Design review of the part built by this model. Coordinates are the model's own, in mm. A direction names the side the tool comes from. Coordinates: 2 decimals unless noted, no trailing zeros. Write each loop counter-clockwise with the first axis right and the second up, starting at its lowest first coordinate (ties: lowest second). Pieces come first, ordered by that corner, then holes. Notation, with made-up numbers: (-13, 17) -> (43, 17) arc R37 cw to (43, 56) -> close; hole circle Ø5 at (39, 8.5). An arc over 180 degrees is marked (long way). Answer in a Markdown table with one row per item. Add a question column.
Item 1: Take a section at B-B, the plane x = -2.5. Write out the cut boundary in (y, z), and give its area (3 significant figures).
Item 2: Take a section at D-D, the plane y = 23. Write out the cut boundary in (x, z), and give its area (3 significant figures).
Item 3: Take a section at A-A, the plane y = 38. Give the number of separate pieces and of enclosed holes in the cut face, and give its area (3 significant figures).
Item 4: To check wall thickness, follow line 1 (Z direction, x = 13.5, y = 36); line 2 (Y direction, x = -2.5, z = -1.65); line 3 (X direction, y = 32, z = -53). State the ranges of each line that lie inside material, in increasing order.
Item 5: Draft analysis for pull direction Z (two halves, no side actions). For faces 4 (the face through (15, 24, 0)), 5 (the face through (19.3, 35.1, -143.9)), 6 (the face through (-2.33, 39.29, -1.52)), state which applies: released by +Z, released by -Z, zero draft, split by the parting line, or undercut.
Item 6: For faces 1 (the face through (15, 20, -92)), 2 (the face through (15, 30, -97)), 3 (the face through (15, 30, -87)), list the 3-axis set-ups (+Z, -Z, +X, -X, +Y, -Y) from which the entire face can be reached by the end or side of a thin tool; tool diameter is ignored.
Item 7: Take a section at C-C, the plane z = -42. Write out the cut boundary in (x, y).
Item 8: Clearance check with flat-ended pins moving along their axes: P1, Ø16, axis at y = 28.5, z = -86.5, coming from the -X side; P2, Ø1.4, axis at x = 20, z = -142.92, coming from the +Y side; P3, Ø1.5, axis at x = -2, y = 31, coming from the -Z side. State where each tip first meets the part, or that it passes through.
from build123d import *

# Parameters (mm, degrees)
SKETCH1_W               = 30
SKETCH1_H               = 150
BOSS_EXTRUDE1_DEPTH     = 40
CUT_EXTRUDE1_DEPTH      = 159.113883008
CUT_EXTRUDE1_DEPTH_BACK = 30
SKETCH2_W               = 22
SKETCH2_H               = 43
SKETCH4_W               = 22
SKETCH4_H               = 10
CUT_EXTRUDE2_DEPTH      = 20
CUT_EXTRUDE3_DEPTH      = 159.113883008
CUT_EXTRUDE3_DEPTH_BACK = 159.113883008
SKETCH5_W               = 150
SKETCH5_H               = 8
SKETCH6_R               = 1.2
CUT_EXTRUDE4_DEPTH      = 10
SKETCH7_W               = 40
SKETCH7_H               = 32
BOSS_EXTRUDE2_DEPTH     = 3
SKETCH8_R               = 1.3
CUT_EXTRUDE5_DEPTH      = 157.31378698
SKETCH9_W               = 22
SKETCH9_H               = 80
CUT_EXTRUDE6_DEPTH      = 158.318148985


with BuildPart() as part:
    # Sketch1 → Boss-Extrude1 (new body)
    with BuildSketch(Plane(origin=(0, 0, 0), x_dir=(1, 0, 0), z_dir=(0, 1, 0))):
        with Locations((15, 75)):
            Rectangle(SKETCH1_W, SKETCH1_H)
    extrude(amount=BOSS_EXTRUDE1_DEPTH)

    # Sketch2 → Cut-Extrude1 (cut, two sides: drawn at the far end of the back side and taken through both)
    with BuildSketch(Plane(origin=(0, 40, 0), x_dir=(1, 0, 0), z_dir=(0, 1, 0)).offset(-CUT_EXTRUDE1_DEPTH_BACK)):
        with Locations((15, 118.5)):
            Rectangle(SKETCH2_W, SKETCH2_H)
    extrude(amount=CUT_EXTRUDE1_DEPTH + CUT_EXTRUDE1_DEPTH_BACK, mode=Mode.SUBTRACT)

    # Sketch4 → Cut-Extrude2 (cut)
    with BuildSketch(Plane.XZ):
        with Locations((15, -92)):
            Rectangle(SKETCH4_W, SKETCH4_H)
    extrude(amount=-CUT_EXTRUDE2_DEPTH, mode=Mode.SUBTRACT)

    # Sketch5 → Cut-Extrude3 (cut, two sides: drawn at the far end of the back side and taken through both)
    with BuildSketch(Plane.ZY.offset(-CUT_EXTRUDE3_DEPTH_BACK)):
        with Locations((-75, 4)):
            Rectangle(SKETCH5_W, SKETCH5_H)
    extrude(amount=CUT_EXTRUDE3_DEPTH + CUT_EXTRUDE3_DEPTH_BACK, mode=Mode.SUBTRACT)

    # Sketch6 → Cut-Extrude4 (cut)
    with BuildSketch(Plane(origin=(0, 40, 0), x_dir=(1, 0, 0), z_dir=(0, 1, 0))):
        with Locations(Location((10, 142.924700648, 0), (0, 0, 270))):
            Circle(SKETCH6_R)
        with Locations(Location((20, 142.924700648, 0), (0, 0, 270))):
            Circle(SKETCH6_R)
        with Locations(Location((10, 94.924700648, 0), (0, 0, 270))):
            Circle(SKETCH6_R)
        with Locations(Location((20, 94.924700648, 0), (0, 0, 270))):
            Circle(SKETCH6_R)
    extrude(amount=-CUT_EXTRUDE4_DEPTH, mode=Mode.SUBTRACT)

    # Sketch7 → Boss-Extrude2 (add)
    with BuildSketch(Plane.XY):
        with Locations((15, 24)):
            Rectangle(SKETCH7_W, SKETCH7_H)
    extrude(amount=-BOSS_EXTRUDE2_DEPTH)

    # Sketch8 → Cut-Extrude5 (cut, through all)
    with BuildSketch(Plane(origin=(0, 0, -3), x_dir=(-1, 0, 0), z_dir=(0, 0, -1))):
        with Locations((-32.5, 38)):
            Circle(SKETCH8_R)
        with Locations((-32.5, 10)):
            Circle(SKETCH8_R)
        with Locations((2.5, 38)):
            Circle(SKETCH8_R)
        with Locations((2.5, 10)):
            Circle(SKETCH8_R)
    extrude(amount=-CUT_EXTRUDE5_DEPTH, mode=Mode.SUBTRACT)

    # Sketch9 → Cut-Extrude6 (cut, through all)
    with BuildSketch(Plane(origin=(0, 40, 0), x_dir=(1, 0, 0), z_dir=(0, 1, 0))):
        with Locations((15, 47)):
            Rectangle(SKETCH9_W, SKETCH9_H)
    extrude(amount=-CUT_EXTRUDE6_DEPTH, mode=Mode.SUBTRACT)


solid = part.part
Answers:
| question | item | result |
|---|---|---|
| 1 | outline | (8, -3) -> (8.7, -3) -> (8.7, 0) -> (8, 0) -> close; (11.3, -3) -> (36.7, -3) -> (36.7, 0) -> (11.3, 0) -> close; (39.3, -3) -> (40, -3) -> (40, 0) -> (39.3, 0) -> close |
| 1 | area | 80.4 mm^2 |
| 2 | outline | (-5, -3) -> (0, -3) -> (0, -150) -> (30, -150) -> (30, -3) -> (35, -3) -> (35, 0) -> (-5, 0) -> close; hole (4, -140) -> (26, -140) -> (26, -97) -> (4, -97) -> close; hole (4, -87) -> (26, -87) -> (26, -7) -> (4, -7) -> close |
| 2 | area | 1,820 mm^2 |
| 3 | separate pieces | 3 |
| 3 | enclosed holes | 6 |
| 3 | area | 1,790 mm^2 |
| 4 | line 1 | z = -150 to -140, -97 to -87, -7 to 0 |
| 4 | line 2 | y = 8 to 8.7, 11.3 to 36.7, 39.3 to 40 |
| 4 | line 3 | x = 0 to 4, 26 to 30 |
| 5 | face 4 | released by +Z |
| 5 | face 5 | undercut |
| 5 | face 6 | zero draft |
| 6 | face 1 | -Y |
| 6 | face 2 | +Y |
| 6 | face 3 | +Y, -Y |
| 7 | outline | (0, 8) -> (4, 8) -> (4, 40) -> (0, 40) -> close; (26, 8) -> (30, 8) -> (30, 40) -> (26, 40) -> close |
| 8 | P1 | stops at x = 0 |
| 8 | P2 | stops at y = 30 |
| 8 | P3 | stops at z = -3 |
